Autodesk Inventor part; units mm, degrees
ref_plane "YZ Plane" through (0, 0, 0) normal (1, 0, 0) x (0, 1, 0)
ref_plane "XZ Plane" through (0, 0, 0) normal (0, 1, 0) x (-1, 0, 0)
ref_plane "XY Plane" through (0, 0, 0) normal (0, 0, 1) x (1, 0, 0)
sketch "スケッチ1" plane through (0, 0, 0) normal (0, 1, 0) x (-1, 0, 0)
  line L0 (0, 0) -> (-90, 0)
  line L1 (-90, 0) -> (-90, 50)
  line L2 (0, 50) -> (0, 0)
  line L3 (0, 0) -> (-5, 0)
  line L4 (-5, 0) -> (-5, 50)
  line L5 (-5, 0) -> (-90, 0)
  line L6 (-90, 0) -> (-85, 0)
  line L7 (-85, 0) -> (-85, 50)
  arc A0 (-85, 50) -> (-5, 50) centre (-45, 50) ccw
  line L8 (0, 0) -> (0, 10)
  line L9 (0, 10) -> (-90, 10)
  circle A1 centre (-45, 50) radius 45
  line L10 (-90, 5) -> (0, 5)
  line L11 (-90, 50) -> (-85, 50)
  line L12 (-5, 50) -> (0, 50)
  line L13 (0, 0) -> (-90, 0)
  line L14 (-90, 0) -> (-90, 5)
  line L15 (-90, 5) -> (0, 5)
  line L16 (0, 5) -> (0, 0)
  dimension "d0" = 90
  dimension "d1" = 50
  dimension "d2" = 5
  dimension "d3" = 85
  dimension "d4" = 5
  dimension "d5" = 80
  dimension "d6" = 10
  dimension "d7" = 90
extrude "押し出し1" add sketch "スケッチ1" along normal blind 230 contours L0 L4 L10 L2 | L0 L7 L10 L4 | L10 L4 L9 L2 | L0 L1 L10 L7 | L10 A1 L9 L4 | L9 L4 A1 L2 | L10 L1 L9 L7 | L7 L9 A1 L10 | L9 A1 L4 | A1 L9 | A1 L4 L12 | L9 L1 A1 L7 | L7 A1 L9 | A1 L9 A0 L4 | A1 L7 A0 L9 | L11 L7 A1
sketch "スケッチ2" plane through (0, 0, 0) normal (0, -1, 0) x (1, 0, 0)
  line L0 (0, 0) -> (0, 50)
  line L1 (90, 0) -> (0, 0)
  line L2 (90, 50) -> (90, 0)
  line L3 (85, 50) -> (90, 50)
  arc A0 (5, 50) -> (85, 50) centre (45, 50) ccw
  line L4 (0, 50) -> (5, 50)
  arc A1 (5, 23.467) -> (85, 23.467) centre (45, 50) ccw
  line L5 (0, 5) -> (90, 5)
  line L6 (5, 23.467) -> (5, 5)
  line L7 (85, 23.467) -> (85, 5)
  dimension "d29" = 48
extrude "押し出し2" cut sketch "スケッチ2" against normal blind 225 contours L6 A1 L5 | L5 A1 L7
sketch "スケッチ3" plane through (0, 230, 0) normal (0, 1, 0) x (1, 0, 0)
  arc A0 (85, -50) -> (5, -50) centre (45, -50) ccw
  line L0 (90, -50) -> (90, 0)
  line L1 (0, -50) -> (5, -50)
  arc A1 (85, -50) -> (5, -50) centre (45, -50) ccw
  line L2 (5, -50) -> (85, -50)
extrude "押し出し3" add sketch "スケッチ3" against normal blind 5
sketch "スケッチ4" plane through (90, 0, 50) normal (1, 0, 0) x (0, 0, -1)
  line L0 (0, 0) -> (50, 0)
  line L1 (0, 0) -> (0, 230)
  line L2 (25, 0) -> (25, 65)
  line L3 (25, 65) -> (25, 75)
  line L4 (25, 75) -> (25, 215)
  line L5 (25, 215) -> (25, 225)
  line L6 (0, 65) -> (40, 65)
  line L7 (40, 65) -> (40, 75)
  line L8 (40, 75) -> (0, 75)
  line L9 (0, 75) -> (0, 65)
  line L10 (0, 215) -> (40, 215)
  line L11 (40, 215) -> (40, 225)
  line L12 (40, 225) -> (0, 225)
  line L13 (0, 225) -> (0, 215)
  dimension "d16" = 65
  dimension "d17" = 10
  dimension "d18" = 140
  dimension "d19" = 10
  dimension "d20" = 40
extrude "押し出し4" cut sketch "スケッチ4" against normal blind 90 contours L1 L8 L3 L6 | L3 L8 L7 L6 | L1 L12 L5 L10 | L5 L12 L11 L10
sketch "スケッチ6" plane through (90, 0, 50) normal (1, 0, 0) x (0, 0, -1)
  line L0 (0, 230) -> (50, 230)
  line L1 (50, 230) -> (37.5, 251.6506)
  line L2 (50, 230) -> (110, 230) construction
  line L3 (0, 230) -> (37.5, 251.6506)
  line L4 (0, 230) -> (43.3013, 230) construction
  dimension "d32" = 120
  dimension "d33" = 30
extrude "押し出し6" add sketch "スケッチ6" against normal blind 90
sketch "スケッチ9" plane through (0, 0, 0) normal (-1, 0, 0) x (0, 0, 1)
  line L0 (10, 225) -> (50, 225)
  line L1 (50, 225) -> (50, 230)
  line L2 (50, 230) -> (12.5, 251.6506)
  line L3 (12.5, 251.6506) -> (0, 230)
  line L4 (0, 0) -> (0, 230)
  line L5 (0, 0) -> (50, 0)
  line L6 (50, 0) -> (50, 65)
  line L7 (50, 65) -> (10, 65)
  line L8 (10, 65) -> (10, 75)
  line L9 (10, 75) -> (50, 75)
  line L10 (50, 75) -> (50, 215)
  line L11 (50, 215) -> (10, 215)
  line L12 (10, 215) -> (10, 225)
  line L13 (12.5, 251.6506) -> (0, 230)
  line L14 (0, 230) -> (-132.7906, 0)
  line L15 (0, 145) -> (-49.0748, 145)
  line L16 (0, 115) -> (-66.3953, 115)
  dimension "d45" = 30
sketch "スケッチ10" plane through (0, 0, 0) normal (-1, 0, 0) x (0, 0, 1)
  line L0 (10, 225) -> (50, 225)
  line L1 (50, 225) -> (50, 230)
  line L2 (50, 230) -> (12.5, 251.6506)
  line L3 (12.5, 251.6506) -> (0, 230)
  line L4 (0, 0) -> (0, 230)
  line L5 (0, 0) -> (50, 0)
  line L6 (50, 0) -> (50, 65)
  line L7 (50, 65) -> (10, 65)
  line L8 (10, 65) -> (10, 75)
  line L9 (10, 75) -> (50, 75)
  line L10 (50, 75) -> (50, 215)
  line L11 (50, 215) -> (10, 215)
  line L12 (10, 215) -> (10, 225)
  line L13 (12.5, 251.6506) -> (-87.5, 78.4456)
  line L14 (-87.5, 78.4456) -> (50, 0)
sketch "スケッチ11" plane through (90, 230, 0) normal (0, 0.5, -0.866) x (-1, 0, 0)
  line L0 (0, 25) -> (90, 25)
  line L1 (45, 25) -> (45, 15)
  line L2 (45, 15) -> (60, 15)
  line L3 (60, 15) -> (30, 15)
  point P0 (90, -199.1858)
  dimension "d49" = 10
  dimension "d50" = 15
  dimension "d51" = 30
hole "穴1" at (45, 242.9904, 7.5) at (30, 242.9904, 7.5) at (60, 242.9904, 7.5) direction (0, -0.5, 0.866) diameter 2.5 depth 8 tip angle 118
sketch "スケッチ12" plane through (90, 0, 50) normal (1, 0, 0) x (0, 0, -1)
  line L0 (50, 0) -> (50, 230)
  line L1 (40, 225) -> (40, 215)
  line L2 (0, 215) -> (0, 75)
  line L3 (0, 145) -> (50, 145)
  line L4 (32.5, 175) -> (17.5, 175)
  line L5 (17.5, 175) -> (17.5, 115)
  line L6 (17.5, 115) -> (32.5, 115)
  line L7 (32.5, 115) -> (32.5, 175)
  line L8 (32.5, 175) -> (17.5, 115) construction
  line L9 (17.5, 175) -> (32.5, 115) construction
  line L10 (17.5, 145) -> (32.5, 145)
  line L11 (32.5, 145) -> (32.5, 115)
  line L12 (32.5, 115) -> (17.5, 115)
  line L13 (17.5, 115) -> (17.5, 145)
  point P0 (25, 145)
  dimension "d59" = 15
  dimension "d60" = 60
extrude "押し出し8" cut sketch "スケッチ12" against normal blind 2.5 contours L3 L7 L6 L5
sketch "スケッチ13" plane through (0, 0, 0) normal (-1, 0, 0) x (0, 0, 1)
  line L0 (0, 0) -> (0, 230)
  line L1 (50, 75) -> (50, 215)
  line L2 (50, 145) -> (0, 145)
  line L3 (17.5, 175) -> (32.5, 175)
  line L4 (32.5, 175) -> (32.5, 115)
  line L5 (32.5, 115) -> (17.5, 115)
  line L6 (17.5, 115) -> (17.5, 175)
  line L7 (17.5, 175) -> (32.5, 115) construction
  line L8 (32.5, 175) -> (17.5, 115) construction
  line L9 (17.5, 145) -> (32.5, 145)
  line L10 (32.5, 145) -> (32.5, 115)
  line L11 (32.5, 115) -> (17.5, 115)
  line L12 (17.5, 115) -> (17.5, 145)
  point P0 (25, 145)
  dimension "d63" = 15
  dimension "d64" = 60
extrude "押し出し9" cut sketch "スケッチ13" against normal blind 2.5 contours L4 L5 L6 L2
sketch "スケッチ14" plane through (90, 0, 0) normal (0, 0, -1) x (-1, 0, 0)
  line L0 (90, 0) -> (90, 230)
  line L1 (0, 0) -> (0, 230)
  line L2 (0, 145) -> (90, 145)
  line L3 (37.5, 170) -> (52.5, 170)
  line L4 (52.5, 170) -> (52.5, 120)
  line L5 (52.5, 120) -> (37.5, 120)
  line L6 (37.5, 120) -> (37.5, 170)
  line L7 (37.5, 170) -> (52.5, 120) construction
  line L8 (52.5, 170) -> (37.5, 120) construction
  line L9 (37.5, 145) -> (52.5, 145)
  line L10 (52.5, 145) -> (52.5, 170)
  line L11 (52.5, 170) -> (37.5, 170)
  line L12 (37.5, 170) -> (37.5, 145)
  point P0 (45, 145)
  dimension "d67" = 15
  dimension "d70" = 25
extrude "押し出し10" cut sketch "スケッチ14" against normal blind 5 contours L6 L3 L4 L2
sketch "スケッチ16" plane through (90, 0, 0) normal (0, 0, -1) x (-1, 0, 0)
  line L0 (52.5, 170) -> (52.5, 145)
  line L1 (52.5, 145) -> (37.5, 145)
  line L2 (37.5, 145) -> (37.5, 170)
  line L3 (90, 0) -> (90, 230)
  line L4 (0, 0) -> (0, 230)
  line L5 (0, 145) -> (90, 145)
  line L6 (0, 160) -> (37.5, 157.5)
  line L7 (52.5, 157.5) -> (90, 157.5)
  line L8 (18.75, 158.75) -> (18.75, 145)
  line L9 (71.25, 145) -> (71.25, 157.5)
  line L10 (11.25, 175) -> (26.25, 175)
  line L11 (26.25, 175) -> (26.25, 115)
  line L12 (26.25, 115) -> (11.25, 115)
  line L13 (11.25, 115) -> (11.25, 175)
  line L14 (11.25, 175) -> (26.25, 115) construction
  line L15 (26.25, 175) -> (11.25, 115) construction
  line L16 (11.25, 115) -> (26.25, 115)
  line L17 (26.25, 115) -> (26.25, 175)
  line L18 (26.25, 175) -> (11.25, 175)
  line L19 (11.25, 175) -> (11.25, 115)
  line L20 (45, 145) -> (45, 125)
  line L21 (78.75, 175) -> (63.75, 175)
  line L22 (63.75, 115) -> (78.75, 115)
  line L23 (78.75, 175) -> (78.75, 115)
  line L24 (63.75, 115) -> (63.75, 175)
  line L25 (63.75, 175) -> (78.75, 175)
  line L26 (78.75, 175) -> (78.75, 115)
  line L27 (78.75, 115) -> (63.75, 115)
  line L28 (63.75, 115) -> (63.75, 175)
  line L29 (11.25, 115) -> (26.25, 115)
  line L30 (26.25, 115) -> (26.25, 175)
  line L31 (26.25, 175) -> (11.25, 175)
  line L32 (11.25, 175) -> (11.25, 115)
  dimension "d71" = 15
  dimension "d72" = 60
  dimension "d73" = 20
extrude "押し出し11" cut sketch "スケッチ16" against normal blind 3 contours L24 L21 L23 L7 | L7 L9 L5 L24 | L5 L23 L22 L24 | L7 L23 L5 L9 | L11 L12 L13 L5 | L5 L8 L6 L11 | L6 L13 L10 L11 | L5 L13 L6 L8
sketch "スケッチ17" plane through (37.5, 145, 0) normal (0, 1, 0) x (1, 0, 0)
  line L0 (-57.7643, 16.522) -> (69.053, 16.522)
  line L1 (69.053, 16.522) -> (69.053, -65.9751)
  line L2 (69.053, -65.9751) -> (-57.7643, -65.9751)
  line L3 (-57.7643, -65.9751) -> (-57.7643, 16.522)
  point P0 (-37.5, 0)
extrude "押し出し12" cut sketch "スケッチ17" against normal blind 180
sketch "スケッチ18" plane through (0, 215, 10) normal (-1, 0, 0) x (0, 0, 1)
  line L0 (-10, -70) -> (40, -70)
  line L1 (7.5, -40) -> (22.5, -40)
  line L2 (22.5, -40) -> (22.5, -100)
  line L3 (22.5, -100) -> (7.5, -100)
  line L4 (7.5, -100) -> (7.5, -40)
  line L5 (7.5, -40) -> (22.5, -100) construction
  line L6 (22.5, -40) -> (7.5, -100) construction
  point P0 (-10, -215)
  point P1 (15, -70)
  dimension "d78" = 15
  dimension "d79" = 60
extrude "押し出し13" add sketch "スケッチ18" against normal blind 2.5
sketch "スケッチ19" plane through (90, 215, 10) normal (1, 0, 0) x (0, 0, -1)
  line L0 (-40, -70) -> (10, -70)
  line L1 (-22.5, -40) -> (-7.5, -40)
  line L2 (-7.5, -40) -> (-7.5, -100)
  line L3 (-7.5, -100) -> (-22.5, -100)
  line L4 (-22.5, -100) -> (-22.5, -40)
  line L5 (-22.5, -40) -> (-7.5, -100) construction
  line L6 (-7.5, -40) -> (-22.5, -100) construction
  point P0 (10, -215)
  point P1 (-15, -70)
  dimension "d82" = 15
  dimension "d83" = 60
extrude "押し出し14" add sketch "スケッチ19" against normal blind 2.5
properties part number "知能ロボコン発射台２.1" material "ABS プラスチック"
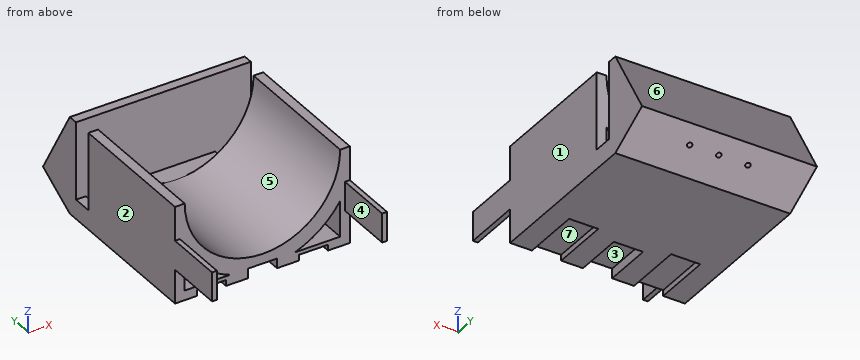
Source: CAD feature listing. Evaluate the final solid. Frame: model axes, mm. Face numbers are marked on the shaded views. A direction names the side the tool comes from. Give positions to 0.01 mm unless a question says otherwise; leave off trailing zeros. Write each loop counter-clockwise with the first axis right and the second up, starting at its lowest first coordinate (ties: lowest second). Pieces come first, ordered by that corner, then holes.
1. First-contact query: pin 1 (1.5 mm diameter, centred on y = 186, z = 42, fed in from -X); pin 2 (0.8 mm diameter, centred on x = 88.5, y = 134.5, fed in from +Z); pin 3 (6 mm diameter, centred on x = 57.5, z = 34.5, fed in from -Y); pin 4 (4 mm diameter, centred on x = 3, y = 222, fed in from +Z). Flat tips, straight axial feed; report the tip coordinate or a pass-through.
2. Material intervals for line 1 along X through (y, z) = (172.5, 16); line 2 along X through (y, z) = (192, 48.5); line 3 along X through (y, z) = (205, 38.5), sorted ascending.
3. Access query for the marked faces 4, 5, 6 and 7. Directions: +Z, -Z, +X, -X, +Y, -Y. A direction counts if a zero-diameter tool reaches every point of the face in a straight line with its end or side. Return the directions, or none.
4. Section query D-D (y = 221.5). Return the cut outline in (x, z).
5. Section query B-B (z = 25). Return the cut outline in (x, y), then the cut area to 3 significant figures.
6. Section query C-C (x = 54). Return the cut outline in (y, z), then the cut area to 3 significant figures.
7. Section query A-A (y = 183.5). Return the cut outline in (x, z), then the cut area to 3 significant figures.
8. Pull-direction query (X, two-part tool) for the marked faces 1, 2 and 3; classes: +X half, -X half, draft (parallel to the pull), parting line (faces both ways), or undercut.
Output values:
1. pin 1: stops at x = 0
1. pin 2: stops at z = 32.5
1. pin 3: stops at y = 225
1. pin 4: stops at z = 10
2. line 1: x = 0 to 5, 11.12 to 23.93, 66.07 to 78.88, 85 to 90
2. line 2: x = 0 to 5.03, 84.97 to 90
2. line 3: x = 0 to 6.69, 83.31 to 90
3. face 4: +Z, -Z, -Y
3. face 5: +Z, -Y
3. face 6: +Z, +X, -X, +Y
3. face 7: -Z, -Y
4. outline: (0, 0) - (90, 0) - (90, 10) - (85, 10) - (85, 5) - (61.7, 5) arc R48 ccw to (71.53, 10) - (18.47, 10) arc R48 ccw to (28.3, 5) - (5, 5) - (5, 10) - (0, 10) - close
5. outline: (0, 115) - (2.5, 115) - (2.5, 145) - (13.78, 145) - (13.78, 215) - (0, 215) - close; (0, 225) - (90, 225) - (90, 244.43) - (0, 244.43) - close; (76.22, 145) - (87.5, 145) - (87.5, 115) - (90, 115) - (90, 215) - (76.22, 215) - close
5. area: 3,830 mm2
6. outline: (145, 0) - (230, 0) - (251.65, 12.5) - (230, 50) - (225, 50) - (225, 10) - (215, 10) - (215, 11.03) - (145, 11.03) - close
6. area: 1,660 mm2
7. outline: (0, 0) - (90, 0) - (90, 50) - (85, 50) arc R40 cw to (5, 50) - (0, 50) - close; hole (5, 5) - (28.3, 5) arc R48 cw to (5, 23.47) - close; hole (61.7, 5) - (85, 5) - (85, 23.47) arc R48 cw to start
7. area: 1,650 mm2
8. face 1: +X half
8. face 2: -X half
8. face 3: undercut
